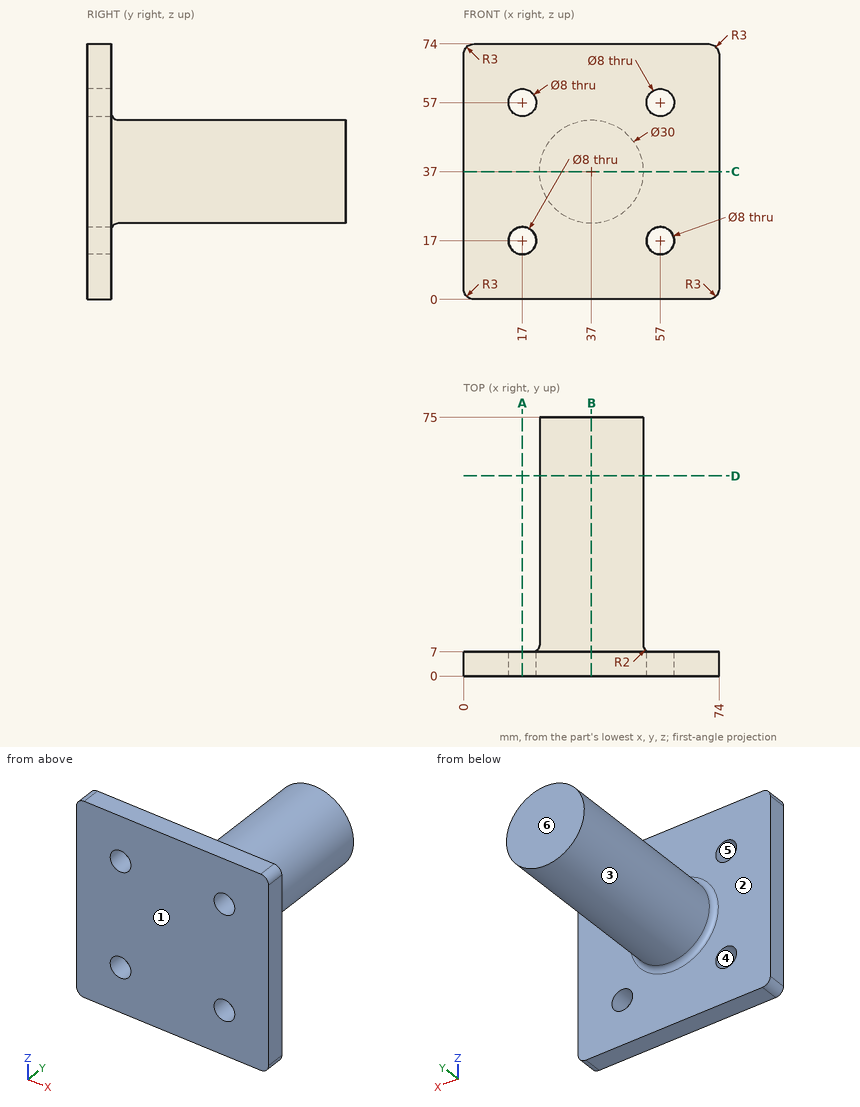
Verification items for this drawing (mm, ordinates from the low corner). A direction names the side the tool comes from. Give positions to 0.01 mm unless a question says otherwise; leave off trailing zeros. Write each loop counter-clockwise with the first axis right and the second up, starting at its lowest first coordinate (ties: lowest second). Pieces come first, ordered by that corner, then holes.
1) Access from +Z, -Z, +X, -X, +Y, -Y to the whole of each face (thin tool, end or side, straight path). Record for the marked faces 1 and 2.
2) Section check C-C, the plane z = 37. Record the boundary of the cut face in (x, y), and give its area (3 significant figures).
3) Section check D-D, the plane y = 58. Record the boundary of the cut face in (x, z).
4) Section check B-B, the plane x = 37. Record the boundary of the cut face in (y, z).
5) Gauge pin test, flat ends, axial feed: pin 1 (6.5 mm diameter, centred on x = 57, z = 57, fed in from +Y); pin 2 (9 mm diameter, centred on x = 17, z = 57, fed in from +Y); pin 3 (8 mm diameter, centred on y = 10.5, z = 58.5, fed in from -X); pin 4 (1 mm diameter, centred on x = 25, y = 67, fed in from -Z). Record the tip position at first contact, or that the pin passes through.
6) Section check A-A, the plane x = 17. Record the boundary of the cut face in (y, z).
7) Material ranges on L1, parallel to X at y = 1, z = 17; L2, parallel to Y at x = 64, z = 24.5; L3, parallel to Z at x = 15.5, y = 4, recorded low to high.
8) Release check for a two-part mould opening along X. For the marked faces 3, 4, 5 and 6 record: pulls with the +X half, pulls with the -X half, needs draft (parallel to the pull), parting line crosses it, or undercut.
Computed:
1. face 1: +Z, -Z, +X, -X, -Y
1. face 2: +Y
2. outline: (0, 0) - (74, 0) - (74, 7) - (54, 7) arc R2 cw to (52, 9) - (52, 75) - (22, 75) - (22, 9) arc R2 cw to (20, 7) - (0, 7) - close
2. area: 2,560 mm2
3. outline: circle Ø30 at (37, 37)
4. outline: (0, 0) - (7, 0) - (7, 20) arc R2 cw to (9, 22) - (75, 22) - (75, 52) - (9, 52) arc R2 cw to (7, 54) - (7, 74) - (0, 74) - close
5. pin 1: passes through
5. pin 2: stops at y = 7
5. pin 3: stops at x = 0
5. pin 4: stops at z = 27.37
6. outline: (0, 0) - (7, 0) - (7, 13) - (0, 13) - close; (0, 21) - (7, 21) - (7, 53) - (0, 53) - close; (0, 61) - (7, 61) - (7, 74) - (0, 74) - close
7. L1: x = 0 to 13, 21 to 53, 61 to 74
7. L2: y = 0 to 7
7. L3: z = 0 to 13.29, 20.71 to 53.29, 60.71 to 74
8. face 3: parting line crosses it
8. face 4: undercut
8. face 5: undercut
8. face 6: needs draft
